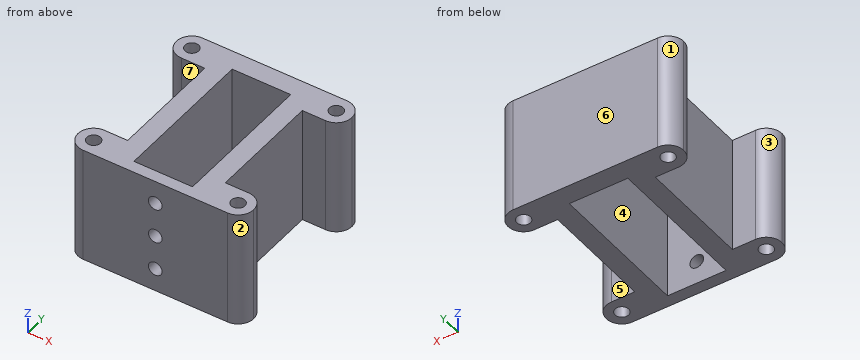
from build123d import *

# Parameters (mm, degrees)
CROQUIS3_W               = 25
CROQUIS3_H               = 45
CROQUIS3_W_2             = 15
CROQUIS3_H_2             = 37
SALIENTE_EXTRUIR1_DEPTH  = 30
CROQUIS4_W               = 30
CROQUIS4_H               = 8
SALIENTE_EXTRUIR2_DEPTH  = 10
CROQUIS5_R               = 1.75
CORTAR_EXTRUIR1_DEPTH    = 49.567948266
REDONDEO1_R              = 4
REDONDEO1_OF_SIMETR_A1_R = 4
CROQUIS7_R               = 1.75
CORTAR_EXTRUIR2_DEPTH    = 59.25672149


with BuildPart() as part:
    # Croquis3 → Saliente-Extruir1 (new body)
    with BuildSketch(Plane.XY):
        with Locations((-4.515654699, -4.5)):
            Rectangle(CROQUIS3_W, CROQUIS3_H)
        with Locations((-4.515654699, -5.5)):
            Rectangle(CROQUIS3_W_2, CROQUIS3_H_2, mode=Mode.SUBTRACT)
    extrude(amount=SALIENTE_EXTRUIR1_DEPTH)

    # Croquis4 → Saliente-Extruir2 (add)
    with BuildSketch(Plane.ZY.offset(17.015654699)):
        with Locations((15, 14)):
            Rectangle(CROQUIS4_W, CROQUIS4_H)
        with Locations((15, -23)):
            Rectangle(CROQUIS4_W, CROQUIS4_H)
    saliente_extruir2 = extrude(amount=SALIENTE_EXTRUIR2_DEPTH)

    # Croquis5 → Cortar-Extruir1 (cut, symmetric)
    with BuildSketch(Plane.XY.offset(30)):
        with Locations((-23.015654699, 14)):
            Circle(CROQUIS5_R)
        with Locations((-23.015654699, -23)):
            Circle(CROQUIS5_R)
    cortar_extruir1 = extrude(amount=CORTAR_EXTRUIR1_DEPTH, both=True, mode=Mode.SUBTRACT)

    # Redondeo1
    redondeo1_edges = [part.edges().sort_by_distance(p)[0] for p in [
        (-27.015654699, -27, 15),
        (-27.015654699, -19, 15),
        (-27.015654699, 10, 15),
        (-27.015654699, 18, 15),
    ]]
    fillet(redondeo1_edges, radius=REDONDEO1_R - 0.0001)  # a hair under: the kernel refuses the full size

    # Simetría1: Saliente-Extruir2, Cortar-Extruir1 across plane
    add(saliente_extruir2.mirror(Plane.ZY.offset(4.515654699)))
    add(cortar_extruir1.mirror(Plane.ZY.offset(4.515654699)), mode=Mode.SUBTRACT)

    # Redondeo1 of Simetría1
    redondeo1_of_simetr_a1_edges = [part.edges().sort_by_distance(p)[0] for p in [
        (17.984345301, -27, 15),
        (17.984345301, -19, 15),
        (17.984345301, 10, 15),
        (17.984345301, 18, 15),
    ]]
    fillet(redondeo1_of_simetr_a1_edges, radius=REDONDEO1_OF_SIMETR_A1_R - 0.0001)  # a hair under: the kernel refuses the full size

    # Croquis7 → Cortar-Extruir2 (cut, through all)
    with BuildSketch(Plane(origin=(0, -24, 0), x_dir=(1, 0, 0), z_dir=(0, 1, 0))):
        with Locations(Location((-4.515654699, -24, 0), (0, 0, 270))):
            Circle(CROQUIS7_R)
        with Locations(Location((-4.515654699, -15, 0), (0, 0, 270))):
            Circle(CROQUIS7_R)
        with Locations(Location((-4.515654699, -6, 0), (0, 0, 270))):
            Circle(CROQUIS7_R)
    extrude(amount=-CORTAR_EXTRUIR2_DEPTH, mode=Mode.SUBTRACT)


solid = part.part
For this review, take the finished solid that the model builds, in its own axes (mm). Face numbers are marked on the shaded views. A direction names the side the tool comes from. Give positions to 0.01 mm unless a question says otherwise; leave off trailing zeros. Loops run counter-clockwise (first coordinate to the right, second up) from the corner with the lowest first, then second, coordinate; pieces in that order, holes last. Notation, with made-up numbers: M 41.5,-6 L 48.5,-6 A18 cw 48.5,17 Z; hole C 45.5,47 d9. An arc over 180 degrees is marked long. Put each result on its own line as item: value. Start each with the question number.
(1) Add section C-C, the plane y = 8. Write out the cut boundary in (x, z).
(2) Machinability: for the marked faces 4, 5, 6 and 7, which of the approach directions +Z, -Z, +X, -X, +Y, -Y give a long, thin tool a straight path to every point of the face, cutting with its end or side? Answer none if there is none.
(3) Add section A-A, the plane x = 1. Write out the cut boundary in (y, z), then the cut area to 3 significant figures.
(4) Wall thickness on L1, parallel to Y at x = 9, z = 20.75; L2, parallel to Y at x = -1, z = 9; L3, parallel to Y at x = 13, z = 19: over which ranges is each line inside the solid? List them lowest first.
(5) For pin 1 (15 mm diameter, centred on y = -14.5, z = 15.5, fed in from +X); pin 2 (2 mm diameter, centred on x = 13.98, y = -23, fed in from +Z); pin 3 (8.5 mm diameter, centred on y = -10, z = 15.5, fed in from +X); pin 4 (1.5 mm diameter, centred on y = 13, z = 20, fed in from -X), all flat-tipped, find the tip position at first contact; note any pin that passes through.
(6) The part is to be moulded in two halves that separate along Y. For the marked faces 1, 2 and 3, say which applies: +Y half, -Y half, draft (parallel to the pull), parting line (faces both ways), or undercut.
(7) Add section D-D, the plane x = 15. Write out the cut boundary in (y, z).
(8) Add section B-B, the plane z = 6. Give the number of separate pieces and of enclosed holes in the cut face, then the cut area to 3 significant figures.
Result:
1. outline: M -17.02,0 L -12.02,0 L -12.02,30 L -17.02,30 Z; M 2.98,0 L 7.98,0 L 7.98,30 L 2.98,30 Z
2. face 4: +Z, -Z
2. face 5: +Z, -Z, +X
2. face 6: +Z, -Z, +X, -X, +Y
2. face 7: +Z, -Z, -X
3. outline: M -27,0 L -24,0 L -24,30 L -27,30 Z; M 13,0 L 18,0 L 18,30 L 13,30 Z
3. area: 240 mm^2
4. L1: y = -27 to -19, 10 to 18
4. L2: y = -27 to -24, 13 to 18
4. L3: y = -27 to -24.45, -21.55 to -19, 10 to 12.55, 15.45 to 18
5. pin 1: stops at x = 17.86
5. pin 2: passes through
5. pin 3: stops at x = 7.98
5. pin 4: stops at x = -27.01
6. face 1: +Y half
6. face 2: -Y half
6. face 3: undercut
7. outline: M -26.87,0 L -24.43,0 L -24.43,30 L -26.87,30 Z; M -21.57,0 L -19.13,0 L -19.13,30 L -21.57,30 Z; M 10.13,0 L 12.57,0 L 12.57,30 L 10.13,30 Z; M 15.43,0 L 17.87,0 L 17.87,30 L 15.43,30 Z
8. separate pieces: 1
8. enclosed holes: 4
8. area: 814 mm^2
